from build123d import *

# Parameters (mm, degrees)
SKETCH_2_R          = 6
EXTRUDE_1_DEPTH     = 30
SKETCH_2_3_R        = 6
EXTRUDE_2_DEPTH     = 6
EXTRUDE_START       = 31
SKETCH_2_4_R        = 6
EXTRUDE_3_DEPTH     = 1
CUT_EXTRUDE_1_REACH = 44.219
SKETCH_4_R          = 2
CUT_EXTRUDE_2_REACH = 48.015
SKETCH_5_W          = 1
SKETCH_5_H          = 11
SKETCH_5_W_2        = 15
SKETCH_5_H_2        = 1
FILLET_1_R          = 0.5
EXTRUDE_4_DEPTH     = 3


with BuildPart() as part:
    # 草图2 → 凸台-拉伸1 (new body)
    # profile 1 of 2: a face of its own
    with BuildSketch(Plane.XY):
        Polygon((17.1, 18), (17.1, 0), (-17.1, 0), (-17.1, 18), (-7.1, 18), (-4.25, 23), (4.25, 23), (7.1, 18), align=None)
        with Locations((0, 11.5)):
            Circle(SKETCH_2_R, mode=Mode.SUBTRACT)
    # profile 2 of 2: a face of its own
    with BuildSketch(Plane.XY):
        with Locations((0, 11.5)):
            Circle(SKETCH_2_R)
    extrude(amount=EXTRUDE_1_DEPTH)

    # 草图2<3> → 凸台-拉伸2 (add)
    with BuildSketch(Plane.XY):
        with Locations((0, 11.5)):
            Circle(SKETCH_2_3_R)
    extrude(amount=-EXTRUDE_2_DEPTH)

    # 草图2<4> → 凸台-拉伸3 (add)
    with BuildSketch(Plane.XY.offset(EXTRUDE_START)):
        with Locations((0, 11.5)):
            Circle(SKETCH_2_4_R)
    extrude(amount=-EXTRUDE_3_DEPTH)

    # 草图4 → 切除-拉伸1 (cut, up to next)
    with BuildSketch(Plane.XZ, mode=Mode.PRIVATE) as cut_extrude_1_sk1:
        with Locations((11.75, 23.75)):
            Circle(SKETCH_4_R)
    cut_extrude_1_tool1 = extrude(cut_extrude_1_sk1.sketch, amount=-CUT_EXTRUDE_1_REACH, mode=Mode.PRIVATE) & part.part
    # 草图4 → 切除-拉伸1 (cut, up to next)
    with BuildSketch(Plane.XZ, mode=Mode.PRIVATE) as cut_extrude_1_sk2:
        with Locations((11.75, 6.25)):
            Circle(SKETCH_4_R)
    cut_extrude_1_tool2 = extrude(cut_extrude_1_sk2.sketch, amount=-CUT_EXTRUDE_1_REACH, mode=Mode.PRIVATE) & part.part
    # 草图4 → 切除-拉伸1 (cut, up to next)
    with BuildSketch(Plane.XZ, mode=Mode.PRIVATE) as cut_extrude_1_sk3:
        with Locations((-11.75, 23.75)):
            Circle(SKETCH_4_R)
    cut_extrude_1_tool3 = extrude(cut_extrude_1_sk3.sketch, amount=-CUT_EXTRUDE_1_REACH, mode=Mode.PRIVATE) & part.part
    # 草图4 → 切除-拉伸1 (cut, up to next)
    with BuildSketch(Plane.XZ, mode=Mode.PRIVATE) as cut_extrude_1_sk4:
        with Locations((-11.75, 6.25)):
            Circle(SKETCH_4_R)
    cut_extrude_1_tool4 = extrude(cut_extrude_1_sk4.sketch, amount=-CUT_EXTRUDE_1_REACH, mode=Mode.PRIVATE) & part.part
    add(cut_extrude_1_tool1.solids().sort_by_distance((11.75, 0, 23.75))[0], mode=Mode.SUBTRACT)
    add(cut_extrude_1_tool2.solids().sort_by_distance((11.75, 0, 6.25))[0], mode=Mode.SUBTRACT)
    add(cut_extrude_1_tool3.solids().sort_by_distance((-11.75, 0, 23.75))[0], mode=Mode.SUBTRACT)
    add(cut_extrude_1_tool4.solids().sort_by_distance((-11.75, 0, 6.25))[0], mode=Mode.SUBTRACT)

    # 草图5 → 切除-拉伸2 (cut, up to next)
    with BuildSketch(Plane.XY.offset(30), mode=Mode.PRIVATE) as cut_extrude_2_sk1:
        with Locations((16.6, 12.5)):
            Rectangle(SKETCH_5_W, SKETCH_5_H)
    cut_extrude_2_tool1 = extrude(cut_extrude_2_sk1.sketch, amount=-CUT_EXTRUDE_2_REACH, mode=Mode.PRIVATE) & part.part
    # 草图5 → 切除-拉伸2 (cut, up to next)
    with BuildSketch(Plane.XY.offset(30), mode=Mode.PRIVATE) as cut_extrude_2_sk2:
        with Locations((-16.6, 12.5)):
            Rectangle(SKETCH_5_W, SKETCH_5_H)
    cut_extrude_2_tool2 = extrude(cut_extrude_2_sk2.sketch, amount=-CUT_EXTRUDE_2_REACH, mode=Mode.PRIVATE) & part.part
    # 草图5 → 切除-拉伸2 (cut, up to next)
    with BuildSketch(Plane.XY.offset(30), mode=Mode.PRIVATE) as cut_extrude_2_sk3:
        with Locations((0, 0.5)):
            Rectangle(SKETCH_5_W_2, SKETCH_5_H_2)
    cut_extrude_2_tool3 = extrude(cut_extrude_2_sk3.sketch, amount=-CUT_EXTRUDE_2_REACH, mode=Mode.PRIVATE) & part.part
    add(cut_extrude_2_tool1.solids().sort_by_distance((16.6, 12.5, 30))[0], mode=Mode.SUBTRACT)
    add(cut_extrude_2_tool2.solids().sort_by_distance((-16.6, 12.5, 30))[0], mode=Mode.SUBTRACT)
    add(cut_extrude_2_tool3.solids().sort_by_distance((0, 0.5, 30))[0], mode=Mode.SUBTRACT)

    # 圆角1
    fillet_1_edges = [part.edges().sort_by_distance(p)[0] for p in [
        (17.1, 0, 15),
        (7.5, 0, 15),
        (-7.5, 0, 15),
        (-17.1, 0, 15),
        (-17.1, 7, 15),
        (-16.1, 7, 15),
        (-16.1, 18, 15),
        (17.1, 7, 15),
        (16.1, 7, 15),
        (16.1, 18, 15),
        (-7.1, 18, 15),
        (7.1, 18, 15),
        (-4.25, 23, 15),
        (4.25, 23, 15),
    ]]
    fillet(fillet_1_edges, radius=FILLET_1_R - 0.0001)  # a hair under: the kernel refuses the full size

    # 草图6 → 凸台-拉伸4 (add)
    with BuildSketch(Plane.XY.offset(31)):
        Polygon((-3, 16.696152423), (3, 16.696152423), (6, 11.5), (3, 6.303847577), (-3, 6.303847577), (-6, 11.5), align=None)
    extrude(amount=EXTRUDE_4_DEPTH)


solid = part.part
The model under review builds one solid part; all positions refer to its coordinate system, in mm. A direction names the side the tool comes from. Coordinates: 2 decimals unless noted, no trailing zeros. Write each loop counter-clockwise with the first axis right and the second up, starting at its lowest first coordinate (ties: lowest second). Pieces come first, ordered by that corner, then holes. Notation, with made-up numbers: M 47,73 L 101,73 A16 ccw 101,82 Z; hole C 80.25,36.5 d2. An arc over 180 degrees is marked long. Put each result on its own line as item: value.
1) Draft analysis for pull direction X (two halves, no side actions). For faces 1 (the cylindrical face through (10.163, 8.874, 22.533)), 2 (the flat face through (5, 9, 31)), 3 (the flat face through (-16.1, 12, 15)), state which applies: released by +X, released by -X, zero draft, split by the parting line, or undercut.
Computed:
face 1: undercut
face 2: zero draft
face 3: released by -X
2) Wall thickness on probe 1 along Z at (x, y) = (11.75, 11.75); probe 2 along Y at (x, z) = (-2, 4.5); probe 3 along Z at (x, y) = (10, 11): over which ranges is each line inside the solid? List them lowest first. Write a range as [from, to].
Computed:
probe 1: z = [0, 4.25], [8.25, 21.75], [25.75, 30]
probe 2: y = [1, 23]
probe 3: z = [0, 5.28], [7.22, 22.78], [24.72, 30]
3) For faces 4 (the cylindrical face through (-1.301, 5.643, 30.507)), 5 (the flat face through (0, 1, 15)), 6 (the flat face through (-5, 9, 31)), 7 (the flat face through (16.1, 12, 15)), list the 3-axis set-ups (+Z, -Z, +X, -X, +Y, -Y) from which the entire face can be reached by the end or side of a thin tool; tool diameter is ignored.
Computed:
face 4: +Z
face 5: +Z, -Z, -Y
face 6: +Z, -X, -Y
face 7: +Z, -Z, +X, +Y
4) Add section A-A on x = 11.75. Give the boundary of the cut face in (y, z).
Computed:
outline: M 0,0 L 18,0 L 18,4.25 L 0,4.25 Z; M 0,8.25 L 18,8.25 L 18,21.75 L 0,21.75 Z; M 0,25.75 L 18,25.75 L 18,30 L 0,30 Z
5) Clearance check with flat-ended pins moving along their axes: pin 1 Ø8 at (y, z) = (12, 10.5) entering from -X; pin 2 Ø6.5 at (x, z) = (11.75, 23.75) entering from +Y; pin 3 Ø2.5 at (x, z) = (-11.75, 6.25) entering from +Y; pin 4 Ø0.9 at (x, z) = (0, 32) entering from -Y. State where each tip first meets the part, or that it passes through.
Computed:
pin 1: stops at x = -16.1
pin 2: stops at y = 18
pin 3: passes through
pin 4: stops at y = 6.3
6) Add section D-D on z = 6.25. State how many separate pieces and enclosed holes the cut face has, then the cut area to 3 significant figures.
Computed:
separate pieces: 3
enclosed holes: 0
area: 491 mm2
7) Add section C-C on y = 9.5. Give the boundary of the cut face in (x, z), then the cut area to 3 significant figures.
Computed:
outline: M -16.1,0 L -5.66,0 L -5.66,-6 L 5.66,-6 L 5.66,0 L 16.1,0 L 16.1,30 L 5.66,30 L 5.66,31 L 4.85,31 L 4.85,34 L -4.85,34 L -4.85,31 L -5.66,31 L -5.66,30 L -16.1,30 Z; hole C -11.75,6.25 d4; hole C -11.75,23.75 d4; hole C 11.75,6.25 d4; hole C 11.75,23.75 d4
area: 1,020 mm2
